from build123d import *

# Parameters (mm, degrees)
SKETCH1_W           = 50.8
SKETCH1_H           = 50.8
BOSS_EXTRUDE1_DEPTH = 5.08
CUT_EXTRUDE1_DEPTH  = 50.8
FILLET1_R           = 25.4


with BuildPart() as part:
    # Sketch1 → Boss-Extrude1 (new body)
    with BuildSketch(Plane(origin=(0, 0, 0), x_dir=(1, 0, 0), z_dir=(0, 1, 0))):
        Rectangle(SKETCH1_W, SKETCH1_H)
    extrude(amount=BOSS_EXTRUDE1_DEPTH)

    # Sketch6 → Cut-Extrude1 (cut)
    with BuildSketch(Plane(origin=(0, 5.08, 0), x_dir=(1, 0, 0), z_dir=(0, 1, 0))):
        Polygon((-25.4, -12.7), (-25.4, 25.4), (12.7, 25.4), align=None)
        Polygon((25.4, 12.7), (25.4, -25.4), (-12.7, -25.4), align=None)
    extrude(amount=-CUT_EXTRUDE1_DEPTH, mode=Mode.SUBTRACT)

    # Fillet1
    fillet1_edges = [part.edges().sort_by_distance(p)[0] for p in [
        (-12.7, 2.54, 25.4),
        (25.4, 2.54, -12.7),
    ]]
    fillet(fillet1_edges, radius=FILLET1_R)


solid = part.part
Read the model definition and answer for the solid it produces. Units are mm, in the model's axes. Give positions to 0.01 mm unless a question says otherwise; leave off trailing zeros. Write each loop counter-clockwise with the first axis right and the second up, starting at its lowest first coordinate (ties: lowest second). Pieces come first, ordered by that corner, then holes. Notation, with made-up numbers: (35.5, 42.25) - (43.5, 42.25) arc R28 cw to (43.5, 70.25) - close; hole circle Ø7 at (77.5, 12.5). An arc over 180 degrees is marked (long way). Use CSV: the item, a comma, the result in double quotes. Start each with the question number.
(1) Consider line 1 along Z through (x, y) = (12.5, 2.4); line 2 along X through (y, z) = (3.9, 18); line 3 along X through (y, z) = (1.1, 4). Determine where each line is inside the solid, lowest interval first.
(2) Find section B-B (z = 17). Give the vertices of the cut face in (x, y).
(3) Find section C-C (x = 8.5). Give the vertices of the cut face in (y, z), plus the area to 3 significant figures.
(4) Given P1, Ø3, axis at y = 2, z = -19.5, coming from the -X side, flat-ended and moving along its own axis, determine where the tip first touches the part or whether it passes through.
(5) Find section A-A (y = 2.2). Give the vertices of the cut face in (x, z).
Findings below:
1,line 1,"-25.2 to 0.2"
1,line 2,"-25.4 to -5.3"
1,line 3,"-16.7 to 8.7"
2,outline,"(-25.4, 0) - (-4.3, 0) - (-4.3, 5.08) - (-25.4, 5.08) - close"
3,outline,"(0, -21.2) - (5.08, -21.2) - (5.08, 4.2) - (0, 4.2) - close"
3,area,"129 mm2"
4,P1,"x = 5.3"
5,outline,"(-25.4, 12.7) - (12.7, -25.4) - (25.4, -25.4) - (25.4, -23.22) arc R25.4 ccw to (17.96, -5.26) - (-5.26, 17.96) arc R25.4 ccw to (-23.22, 25.4) - (-25.4, 25.4) - close"
